Autodesk Inventor part; units mm, degrees
ref_plane "Work Plane1" through (0, 0, -25.4) normal (0, 0, -1) x (-1, 0, 0)
ref_plane "Work Plane2" through (63.5, 0, 0) normal (1, 0, 0) x (0, 0, -1)
ref_plane "YZ Plane" through (0, 0, 0) normal (1, 0, 0) x (0, 1, 0)
sketch "Sketch2" plane through (0, 0, 0) normal (1, 0, 0) x (0, 1, 0)
  circle A0 centre (0, 0) radius 25.4
  arc A1 (0, 44.45) -> (0, -44.45) centre (0, 0) ccw
  line L0 (0, -44.45) -> (0, 25.4)
  line L1 (0, 44.45) -> (44.45, 44.45)
  line L2 (44.45, 44.45) -> (44.45, -44.45)
  line L3 (44.45, -44.45) -> (0, -44.45)
  dimension "d0" = 50.8
  dimension "d2" = 88.9
  dimension "d3" = 44.45
extrude "Extrusion1" add sketch "Sketch2" along normal blind 127
sketch "Sketch3" plane through (0, 0, 44.45) normal (0, 0, 1) x (1, 0, 0)
  line L0 (0, 0) -> (127, 0)
  line L1 (0, 0) -> (127, 0)
  line L2 (63.5, 0) -> (0, 0)
  line L3 (63.5, 0) -> (127, 0)
  circle A0 centre (31.75, 0) radius 4.2333
  circle A1 centre (95.25, 0) radius 4.2333
  dimension "d6" = 8.4667
  dimension "d7" = 8.4667
hole "Hole1" at (95.25, 0, 44.45) at (31.75, 0, 44.45) direction (0, 0, -1) diameter 6.35 end through all
ref_plane "Work Plane1" through (0, 0, -25.4) normal (0, 0, -1) x (-1, 0, 0)
sketch "Sketch4" plane through (0, 0, -25.4) normal (0, 0, -1) x (-1, 0, 0)
  arc A0 (-92.075, 0) -> (-98.425, 0) centre (-95.25, 0) ccw
  arc A1 (-28.575, 0) -> (-34.925, 0) centre (-31.75, 0) ccw
  line L0 (-95.25, 0) -> (-101.6, 0)
  line L1 (-101.6, 3.6662) -> (-95.25, 7.3323)
  line L2 (-95.25, 7.3323) -> (-88.9, 3.6662)
  line L3 (-88.9, 3.6662) -> (-88.9, -3.6662)
  line L4 (-88.9, -3.6662) -> (-95.25, -7.3323)
  line L5 (-95.25, -7.3323) -> (-101.6, -3.6662)
  line L6 (-101.6, -3.6662) -> (-101.6, 3.6662)
  line L7 (-31.75, 0) -> (-25.4, 0)
  line L8 (-25.4, -3.6662) -> (-31.75, -7.3323)
  line L9 (-31.75, -7.3323) -> (-38.1, -3.6662)
  line L10 (-38.1, -3.6662) -> (-38.1, 3.6662)
  line L11 (-38.1, 3.6662) -> (-31.75, 7.3323)
  line L12 (-31.75, 7.3323) -> (-25.4, 3.6662)
  line L13 (-25.4, 3.6662) -> (-25.4, -3.6662)
  point P0 (0, 0)
  dimension "d15" = 6.35
extrude "Extrusion2" add sketch "Sketch4" along normal blind 6.35
extrude "Extrusion3" cut sketch "Sketch4" against normal blind 57.15
sketch "Sketch5" plane through (0, 0, -44.45) normal (0, 0, -1) x (-1, 0, 0)
  line L0 (-101.6, 3.6662) -> (-95.25, 7.3323)
  line L1 (-95.25, 7.3323) -> (-88.9, 3.6662)
  line L2 (-88.9, 3.6662) -> (-88.9, -3.6662)
  line L3 (-34.925, 0) -> (-92.075, 0)
  line L4 (0, 0) -> (-28.575, 0)
  line L5 (0, 0) -> (0, 0)
  line L6 (0, 0) -> (-28.575, 0)
  line L7 (-34.925, 0) -> (-92.075, 0)
  line L8 (-98.425, 0) -> (-127, 0)
  line L9 (-127, 0) -> (-127, 0)
  line L10 (-98.425, 0) -> (-127, 0)
  line L11 (-88.9, -3.6662) -> (-95.25, -7.3323)
  line L12 (-95.25, -7.3323) -> (-101.6, -3.6662)
  line L13 (-101.6, -3.6662) -> (-101.6, 3.6662)
  line L14 (-38.1, 3.6662) -> (-31.75, 7.3323)
  line L15 (-25.4, -3.6662) -> (-31.75, -7.3323)
  line L16 (-31.75, 7.3323) -> (-25.4, 3.6662)
  line L17 (-25.4, 3.6662) -> (-25.4, -3.6662)
  line L18 (-38.1, -3.6662) -> (-38.1, 3.6662)
  line L19 (-31.75, -7.3323) -> (-38.1, -3.6662)
extrude "Extrusion4" cut sketch "Sketch5" against normal blind 3.175
sketch "Sketch6" plane through (0, 0, 44.45) normal (0, 0, 1) x (1, 0, 0)
  line L0 (25.4, 0) -> (25.4, -3.6662)
  line L1 (25.4, -3.6662) -> (31.75, -7.3323)
  line L2 (31.75, -7.3323) -> (38.1, -3.6662)
  line L3 (38.1, -3.6662) -> (38.1, 0)
  line L4 (38.1, 0) -> (88.9, 0)
  line L5 (88.9, 0) -> (88.9, -3.6662)
  line L6 (88.9, -3.6662) -> (95.25, -7.3323)
  line L7 (95.25, -7.3323) -> (101.6, -3.6662)
  line L8 (101.6, -3.6662) -> (101.6, 0)
  line L9 (101.6, 0) -> (127, 0)
  line L10 (127, 0) -> (127, 0)
  line L11 (98.425, 0) -> (127, 0)
  line L12 (34.925, 0) -> (92.075, 0)
  line L13 (0, 0) -> (28.575, 0)
  line L14 (0, 0) -> (0, 0)
  line L15 (0, 0) -> (25.4, 0)
  line L16 (38.1, 3.6662) -> (31.75, 7.3323)
  line L17 (38.1, -3.6662) -> (38.1, 3.6662)
  line L18 (31.75, 7.3323) -> (25.4, 3.6662)
  line L19 (25.4, 3.6662) -> (25.4, -3.6662)
  line L20 (88.9, 3.6662) -> (88.9, -3.6662)
  line L21 (95.25, 7.3323) -> (88.9, 3.6662)
  line L22 (101.6, 3.6662) -> (95.25, 7.3323)
  line L23 (101.6, -3.6662) -> (101.6, 3.6662)
extrude "Extrusion5" cut sketch "Sketch6" against normal blind 3.175
sketch "Sketch7" plane through (0, 0, -44.45) normal (0, 0, -1) x (-1, 0, 0)
  line L0 (-101.6, 0) -> (-127, 0)
  line L1 (-101.6, 0) -> (-101.6, 3.6662)
  line L2 (-101.6, 3.6662) -> (-95.25, 7.3323)
  line L3 (-95.25, 7.3323) -> (-88.9, 3.6662)
  line L4 (-88.9, 3.6662) -> (-88.9, 0)
  line L5 (-38.1, 0) -> (-88.9, 0)
  line L6 (-95.25, 0) -> (-107.95, 0)
  line L7 (-31.75, 0) -> (-44.45, 0)
  line L8 (-107.95, 7.3323) -> (-95.25, 14.6647)
  line L9 (-95.25, 14.6647) -> (-82.55, 7.3323)
  line L10 (-82.55, 7.3323) -> (-82.55, -7.3323)
  line L11 (-82.55, -7.3323) -> (-95.25, -14.6647)
  line L12 (-95.25, -14.6647) -> (-107.95, -7.3323)
  line L13 (-107.95, -7.3323) -> (-107.95, 7.3323)
  line L14 (-44.45, 7.3323) -> (-31.75, 14.6647)
  line L15 (-31.75, 14.6647) -> (-19.05, 7.3323)
  line L16 (-19.05, 7.3323) -> (-19.05, -7.3323)
  line L17 (-19.05, -7.3323) -> (-31.75, -14.6647)
  line L18 (-31.75, -14.6647) -> (-44.45, -7.3323)
  line L19 (-44.45, -7.3323) -> (-44.45, 7.3323)
  line L20 (-95.25, -7.3323) -> (-88.9, -3.6662)
  line L21 (-88.9, -3.6662) -> (-88.9, 0)
  line L22 (-101.6, -3.6662) -> (-95.25, -7.3323)
  line L23 (-101.6, 0) -> (-101.6, -3.6662)
  circle A0 centre (-31.75, 0) radius 3.175
  line L24 (-38.1, 3.6662) -> (-31.75, 7.3323)
  line L25 (-38.1, -3.6662) -> (-38.1, 3.6662)
  line L26 (-31.75, -7.3323) -> (-38.1, -3.6662)
  line L27 (-25.4, -3.6662) -> (-31.75, -7.3323)
  line L28 (-25.4, 3.6662) -> (-25.4, -3.6662)
  line L29 (-31.75, 7.3323) -> (-25.4, 3.6662)
  dimension "d24" = 12.7
  dimension "d25" = 12.7
extrude "Extrusion6" add sketch "Sketch7" along normal mid plane 6.35 contours L23 L22 L20 L21 L5 L10 L11 L12 L13 L0 | L0 L13 L8 L9 L10 L5 L4 L3 L2 L1 | L19 L14 L15 L16 L17 L18
sketch "Sketch8" plane through (0, 0, 44.45) normal (0, 0, 1) x (1, 0, 0)
  line L0 (101.6, 3.6662) -> (95.25, 7.3323)
  line L1 (95.25, 7.3323) -> (88.9, 3.6662)
  line L2 (88.9, 3.6662) -> (88.9, -3.6662)
  line L3 (88.9, -3.6662) -> (95.25, -7.3323)
  line L4 (95.25, -7.3323) -> (101.6, -3.6662)
  line L5 (101.6, -3.6662) -> (101.6, 3.6662)
  line L6 (107.95, 7.3323) -> (107.95, -7.3323)
  line L7 (107.95, -7.3323) -> (95.25, -14.6647)
  line L8 (95.25, -14.6647) -> (82.55, -7.3323)
  line L9 (82.55, -7.3323) -> (82.55, 7.3323)
  line L10 (82.55, 7.3323) -> (95.25, 14.6647)
  line L11 (95.25, 14.6647) -> (107.95, 7.3323)
  line L12 (31.75, 7.3323) -> (25.4, 3.6662)
  line L13 (25.4, 3.6662) -> (25.4, -3.6662)
  line L14 (25.4, -3.6662) -> (31.75, -7.3323)
  line L15 (31.75, -7.3323) -> (38.1, -3.6662)
  line L16 (38.1, -3.6662) -> (38.1, 3.6662)
  line L17 (38.1, 3.6662) -> (31.75, 7.3323)
  line L18 (44.45, 7.3323) -> (44.45, -7.3323)
  line L19 (44.45, -7.3323) -> (31.75, -14.6647)
  line L20 (31.75, -14.6647) -> (19.05, -7.3323)
  line L21 (19.05, -7.3323) -> (19.05, 7.3323)
  line L22 (19.05, 7.3323) -> (31.75, 14.6647)
  line L23 (31.75, 14.6647) -> (44.45, 7.3323)
extrude "Extrusion7" add sketch "Sketch8" along normal mid plane 6.35
sketch "Sketch11" plane through (0, 0, -44.45) normal (0, 0, -1) x (-1, 0, 0)
  line L0 (-107.95, 0) -> (-107.95, 7.3323)
  line L1 (-107.95, 7.3323) -> (-95.25, 14.6647)
  line L2 (-95.25, 14.6647) -> (-82.55, 7.3323)
  line L3 (-82.55, 7.3323) -> (-82.55, 0)
  line L4 (-44.45, 0) -> (-82.55, 0)
  line L5 (-44.45, 0) -> (-44.45, 7.3323)
  line L6 (-44.45, 7.3323) -> (-31.75, 14.6647)
  line L7 (-31.75, 14.6647) -> (-19.05, 7.3323)
  line L8 (-19.05, 7.3323) -> (-19.05, 0)
  line L9 (0, 0) -> (-19.05, 0)
  line L10 (0, 0) -> (0, 44.45)
  line L11 (0, 44.45) -> (-127, 44.45)
  line L12 (-127, 0) -> (-127, 44.45)
  line L13 (-107.95, 0) -> (-127, 0)
  line L14 (-127, 44.45) -> (0, 44.45)
  line L15 (0, 44.45) -> (0, 19.05)
  line L16 (0, 19.05) -> (-127, 19.05)
  line L17 (-127, 19.05) -> (-127, 44.45)
extrude "Extrusion9" add sketch "Sketch11" along normal blind 50.8 contours L12 L11 L10 L16
ref_plane "Work Plane2" through (63.5, 0, 0) normal (1, 0, 0) x (0, 0, -1)
sketch "Sketch13" plane through (63.5, 0, 0) normal (1, 0, 0) x (0, 0, -1)
  circle A0 centre (0, 0) radius 25.4
  arc A1 (-44.45, 0) -> (44.45, 0) centre (0, 0) ccw
  line L0 (44.45, 0) -> (44.45, 19.05)
  line L1 (44.45, 19.05) -> (95.25, 19.05)
  line L2 (95.25, 44.45) -> (95.25, 19.05)
  line L3 (-44.45, 44.45) -> (95.25, 44.45)
  line L4 (-44.45, 44.45) -> (-44.45, 0)
  line L5 (95.25, 19.05) -> (88.9, 19.05)
  line L6 (88.9, 19.05) -> (29.3739, -33.3613)
  dimension "d65" = 6.35
extrude "Extrusion10" add sketch "Sketch13" along normal mid plane 25.4 contours A1 L0 L1 L6
sketch "Sketch14" plane through (127, 0, 0) normal (1, 0, 0) x (0, 0, -1)
  arc A0 (29.3739, -33.3613) -> (44.45, 0) centre (0, 0) ccw
  line L0 (29.3739, -33.3613) -> (88.9, 19.05)
  line L1 (44.45, 19.05) -> (88.9, 19.05)
  line L2 (44.45, 0) -> (44.45, 19.05)
  circle A1 centre (0, 0) radius 25.4
  arc A2 (-44.45, 0) -> (44.45, 0) centre (0, 0) ccw
  line L3 (44.45, 0) -> (44.45, 19.05)
  line L4 (44.45, 19.05) -> (95.25, 19.05)
  line L5 (95.25, 44.45) -> (95.25, 19.05)
  line L6 (-44.45, 44.45) -> (95.25, 44.45)
  line L7 (-44.45, 44.45) -> (-44.45, 0)
extrude "Extrusion11" add sketch "Sketch14" against normal blind 12.7 contours A0 L2 L1 L0
sketch "Sketch15" plane through (0, 0, 0) normal (-1, 0, 0) x (0, 0, 1)
  arc A0 (-44.45, 0) -> (-29.3739, -33.3613) centre (0, 0) ccw
  line L0 (-44.45, 19.05) -> (-44.45, 0)
  line L1 (-88.9, 19.05) -> (-44.45, 19.05)
  line L2 (-88.9, 19.05) -> (-29.3739, -33.3613)
  circle A1 centre (0, 0) radius 25.4
  arc A2 (-44.45, 0) -> (44.45, 0) centre (0, 0) ccw
  line L3 (44.45, 44.45) -> (44.45, 0)
  line L4 (44.45, 44.45) -> (-95.25, 44.45)
  line L5 (-95.25, 19.05) -> (-95.25, 44.45)
  line L6 (-44.45, 19.05) -> (-95.25, 19.05)
  line L7 (-44.45, 0) -> (-44.45, 19.05)
extrude "Extrusion12" add sketch "Sketch15" against normal blind 12.7 contours A0 L2 L1 L0
sketch "Sketch16" plane through (0, 44.45, 44.45) normal (0, 1, 0) x (1, 0, 0)
  line L0 (0, 0) -> (0, 139.7)
  line L1 (127, 0) -> (127, 139.7)
  line L2 (107.95, 88.9) -> (114.3, 88.9)
  line L3 (107.95, 88.9) -> (95.25, 88.9)
  line L4 (95.25, 88.9) -> (82.55, 88.9)
  line L5 (76.2, 88.9) -> (82.55, 88.9)
  line L6 (76.2, 88.9) -> (114.3, 88.9)
  line L7 (114.3, 88.9) -> (127, 88.9)
  line L8 (127, 88.9) -> (0, 88.9)
  line L9 (0, 88.9) -> (127, 88.9)
  line L10 (127, 88.9) -> (127, 139.7)
  line L11 (127, 139.7) -> (0, 139.7)
  line L12 (0, 139.7) -> (0, 88.9)
  circle A0 centre (63.5, 114.3) radius 6.985
  point P0 (0, 44.45)
  dimension "d72" = 13.97
hole "Hole3" at (63.5, 44.45, -69.85) direction (0, -1, 0) diameter 13.97 end through all
sketch "Sketch17" plane through (63.5, 0, 0) normal (1, 0, 0) x (0, 0, -1)
  line L0 (62.865, 44.45) -> (76.835, 44.45)
  line L1 (62.865, 44.45) -> (43.815, 44.45)
  line L2 (69.85, 44.45) -> (69.85, 57.15)
  line L3 (69.85, 57.15) -> (43.815, 44.45)
  point P0 (0, 0)
  dimension "d81" = 19.05
  dimension "d82" = 12.7
properties part number "bike_gipper"
The listing builds one solid part. Answer for the finished solid, in the listing's coordinates (mm). A direction names the side the tool comes from. Give positions to 0.01 mm unless a question says otherwise; leave off trailing zeros. Loops run counter-clockwise (first coordinate to the right, second up) from the corner with the lowest first, then second, coordinate; pieces in that order, holes last. Notation, with made-up numbers: (89, 54.5) - (139, 54.5) arc R32 ccw to (139, 85.5) - close; hole circle Ø3 at (77.25, 67). An arc over 180 degrees is marked (long way). Answer as a JSON object with one key per item and string values.
1. A cutting plane is placed at D-D (z = -35). Write down the section's boundary in (x, y) (3 decimals), then the cut area to 3 significant figures.
Determined:
{"outline": "(0, -28.408) - (12.7, -28.408) - (12.7, -27.401) - (50.8, -27.401) - (50.8, -28.408) - (76.2, -28.408) - (76.2, -27.401) - (114.3, -27.401) - (114.3, -28.408) - (127, -28.408) - (127, 44.45) - (0, 44.45) - close; hole circle Ø6.35 at (31.75, 0); hole circle Ø6.35 at (95.25, 0)", "area": "9,110 mm²"}
2. Flat-ended cylindrical pins translate along their axes: pin 1 Ø4 at (x, y) = (95, 0) entering from -Z; pin 2 Ø22.5 at (x, z) = (63.5, -69.85) entering from -Y; pin 3 Ø8 at (x, z) = (15.5, 29) entering from -Y. Find the tip coordinate at first contact, or state that the pin passes through.
Determined:
{"pin 1": "z = -31.75", "pin 2": "y = -7.63", "pin 3": "y = -36.75"}
3. A cutting plane is placed at C-C (y = -21). Write down the section's boundary in (x, z), then the cut area to 3 significant figures.
Determined:
{"outline": "(0, -43.41) - (12.7, -43.41) - (12.7, -39.18) - (50.8, -39.18) - (50.8, -43.41) - (76.2, -43.41) - (76.2, -39.18) - (114.3, -39.18) - (114.3, -43.41) - (127, -43.41) - (127, -14.29) - (0, -14.29) - close; (0, 14.29) - (127, 14.29) - (127, 39.18) - (0, 39.18) - close", "area": "6,540 mm²"}
4. For faces 4 (the flat face through (82.55, 0, -46)), 5 (the flat face through (92.825, 5.932, -24.987)), 6 (the flat face through (92.119, 5.525, 44.406)), 7 (the flat face through (88.811, 10.947, 46.015)), determine the directions among +Z, -Z, +X, -X, +Y, -Y from which every point of the face is accessible in a straight line to the end or side of a thin tool.
Determined:
{"face 4": "-Z, -Y", "face 5": "none", "face 6": "+Z", "face 7": "+Z, +Y"}
5. Find the intervals of material crossed by L1, parallel to X at y = 9.5, z = -69.85 (3 decimals); L2, parallel to X at y = 0, z = -34 (3 decimals); L3, parallel to X at y = -2.5, z = -56, in increasing order. Write a range as [from, to].
Determined:
{"L1": "[0, 12.7], [50.8, 56.515], [70.485, 76.2], [114.3, 127]", "L2": "[0, 28.575], [34.925, 92.075], [98.425, 127]", "L3": "[0, 12.7], [50.8, 76.2], [114.3, 127]"}
6. For a pull along Z with two mould halves and no side action, classify faces 1 (the flat face through (98.381, -5.525, 44.406)), 2 (the flat face through (29, -2, 41.275)), 3 (the cylindrical face through (61.4, 25.32, -63.19)) as pulls with the +Z half, pulls with the -Z half, needs draft (parallel to the pull), parting line crosses it, or undercut.
Determined:
{"face 1": "needs draft", "face 2": "pulls with the +Z half", "face 3": "undercut"}
7. A cutting plane is placed at A-A (z = 0). Write down the section's boundary in (x, y), then the cut area to 3 significant figures.
Determined:
{"outline": "(0, -44.45) - (127, -44.45) - (127, -25.4) - (0, -25.4) - close; (0, 25.4) - (127, 25.4) - (127, 44.45) - (0, 44.45) - close", "area": "4,840 mm²"}
8. A cutting plane is placed at B-B (x = 63.5). Write down the section's boundary in (y, z) (3 decimals), then the cut area to 3 significant figures.
Determined:
{"outline": "(-33.361, -29.374) - (-3.873, -62.865) - (44.45, -62.865) - (44.45, 44.45) - (0, 44.45) arc R44.45 ccw to start; (8.427, -76.835) - (19.05, -88.9) - (19.05, -95.25) - (44.45, -95.25) - (44.45, -76.835) - close; hole circle Ø50.8 at (0, 0)", "area": "6,650 mm²"}
